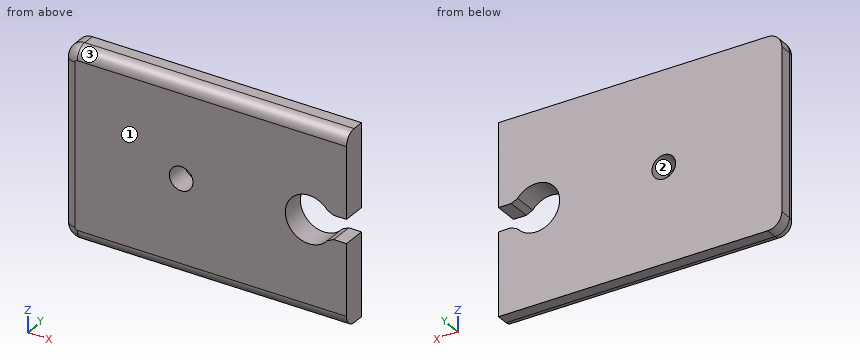
from build123d import *

# Parameters (mm, degrees)
F0_R        = 5
F1_DEPTH    = 10
F2_DEPTH    = 23.2
F3_R        = 6
F4_T1_DEPTH = 19.4160695157
F5_R        = 5


# Not quite as in the source:
# - a fillet or chamfer that OpenCascade refuses, or shapes differently, is made with other operations: its cross-section is extruded or revolved along the edge and cut away or added


with BuildPart() as f1:
    # F0 (on Front) → F1 (new body)
    with BuildSketch(Plane.XZ):
        with BuildLine():
            Line((53.1680434942, 40), (-66.8319565058, 40))
            Line((-66.8319565058, 40), (-66.8319565058, -40))
            Line((-66.8319565058, -40), (53.1680434942, -40))
            Line((53.1680434942, -40), (53.1680434942, -5))
            Line((53.1680434942, -5), (47.2735762596, -5))
            Line((47.2735762596, -5), (45.9338302975, -5))
            ThreePointArc((45.9338302975, -5), (27.2735762596, 0), (45.9338302975, 5))
            Line((45.9338302975, 5), (47.2735762596, 5))
            Line((47.2735762596, 5), (53.1680434942, 5))
            Line((53.1680434942, 5), (53.1680434942, 40))
        make_face()
        with Locations((-16.8319565058, 0)):
            Circle(F0_R, mode=Mode.SUBTRACT)
    extrude(amount=F1_DEPTH)

    # F0 (on Front) → F2 (cut)
    with BuildSketch(Plane.XZ):
        with Locations((-16.8319565058, 0)):
            Circle(F0_R)
    extrude(amount=-F2_DEPTH, mode=Mode.SUBTRACT)

    # F3
    f3_edges = [f1.edges().sort_by_distance(p)[0] for p in [
        (-66.831957, -5, -40),
        (-66.831957, -5, 40),
    ]]
    fillet(f3_edges, radius=F3_R)

    # F4: chamfer of 2 on 2 edges, made by hand

    # F4_s2 → F4_t1 (cut)
    with BuildSketch(Plane.XZ.offset(-4.7080347579)):
        with BuildLine():
            Line((44.9783315762, -6.3208937548), (47.8167286643, -4.9655276174))
            Line((47.8167286643, -4.9655276174), (47.8167286643, -4.9255276174))
            ThreePointArc((47.8167286643, -4.9255276174), (46.8752794809, -4.96), (45.9338302975, -4.96))
            Line((45.9338302975, -4.96), (45.8991892813, -4.98))
            ThreePointArc((45.8991892813, -4.98), (45.4646544727, -5.6663778296), (44.9472237878, -6.2957480693))
            Line((44.9472237878, -6.2957480693), (44.9783315762, -6.3208937548))
        make_face()
        with BuildLine():
            Line((47.8167286643, 4.9655276174), (44.9783315762, 6.3208937548))
            Line((44.9783315762, 6.3208937548), (44.9472237878, 6.2957480693))
            ThreePointArc((44.9472237878, 6.2957480693), (45.4646544727, 5.6663778296), (45.8991892813, 4.98))
            Line((45.8991892813, 4.98), (45.9338302975, 4.96))
            ThreePointArc((45.9338302975, 4.96), (46.8752794809, 4.96), (47.8167286643, 4.9255276174))
            Line((47.8167286643, 4.9255276174), (47.8167286643, 4.9655276174))
        make_face()
    extrude(amount=F4_T1_DEPTH, mode=Mode.SUBTRACT)

    # F5
    f5_edges = [f1.edges().sort_by_distance(p)[0] for p in [
        (-3.831957, -10, -40),
        (-3.831957, -10, 40),
        (-65.074597, -10, 38.242641),
        (-65.074597, -10, -38.242641),
        (-66.831957, -10, 0),
    ]]
    fillet(f5_edges, radius=F5_R)


solid = f1.part
Design review of the part built by this model. Coordinates are the model's own, in mm. Face numbers are marked on the shaded views. Coordinates: 2 decimals unless noted, no trailing zeros. Order: outer loops, then holes, each group sorted by start corner. A loop starts at its lowest first (then second) coordinate and runs counter-clockwise, first axis right, second up.
Item 1: For line 1 (X direction, y = -1, z = -34.5); line 2 (Z direction, x = -59, y = -5.5); line 3 (Z direction, x = 40, y = -2.5), list the stretches that pass through material, from the lowest coordinate up.
Item 2: The part is to be moulded in two halves that separate along Z. For the marked faces 1, 2 and 3, say which applies: pulls with the +Z half, pulls with the -Z half, needs draft (parallel to the pull), parting line crosses it, or undercut.
Item 3: Take a section at A-A, the plane z = 0. Write out the cut boundary in (x, y).
Item 4: Take a section at B-B, the plane y = -2.75. Write out the cut boundary in (x, z), then the cut area to 3 significant figures.
Item 5: Take a section at C-C, the plane x = 29.5. Write out the cut boundary in (y, z), then the cut area to 3 significant figures.
Item 6: For pin 1 Ø9 at (x, z) = (-16.83, 0) entering from +Y; pin 2 Ø1 at (y, z) = (-8.5, -11.5) entering from -X; pin 3 Ø1 at (x, y) = (13, -8) entering from -Z, all flat-tipped, find the tip position at first contact; note any pin that passes through.
The answers:
1. line 1: x = -66.81 to 53.17
1. line 2: z = -39.97 to 39.97
1. line 3: z = -40 to -9.62, 9.62 to 40
2. face 1: needs draft
2. face 2: undercut
2. face 3: pulls with the +Z half
3. outline: (-66.83, -5) arc R5 ccw to (-61.83, -10) - (-21.83, -10) - (-21.83, 0) - (-66.83, 0) - close; (-11.83, -10) - (27.27, -10) - (27.27, 0) - (-11.83, 0) - close
4. outline: (-66.83, -34) arc R6 ccw to (-60.83, -40) - (53.17, -40) - (53.17, -5) - (47.74, -5) - (45.05, -6.29) arc R10 cw (long way) to (45.05, 6.29) - (47.74, 5) - (53.17, 5) - (53.17, 40) - (-60.83, 40) arc R6 ccw to (-66.83, 34) - close; hole circle Ø10 at (-16.83, 0)
4. area: 9,130 mm2
5. outline: (-10, -35) arc R5 ccw to (-5, -40) - (0, -40) - (0, -6.29) - (-10, -6.29) - close; (-10, 6.29) - (0, 6.29) - (0, 40) - (-5, 40) arc R5 ccw to (-10, 35) - close
5. area: 663 mm2
6. pin 1: passes through
6. pin 2: stops at x = -65.83
6. pin 3: stops at z = -39.33
